The drawing under review shows one solid part. Ordinate dimensions are in mm from its lowest x, y, z. Give positions to 0.01 mm unless a question says otherwise; leave off trailing zeros. Write each loop counter-clockwise with the first axis right and the second up, starting at its lowest first coordinate (ties: lowest second). Pieces come first, ordered by that corner, then holes. Notation, with made-up numbers: M 67,8 L 117,8 A16 ccw 117,14 Z; hole C 42.25,30.5 d5. An arc over 180 degrees is marked long. Write item = value, one per line. Start each with the question number.
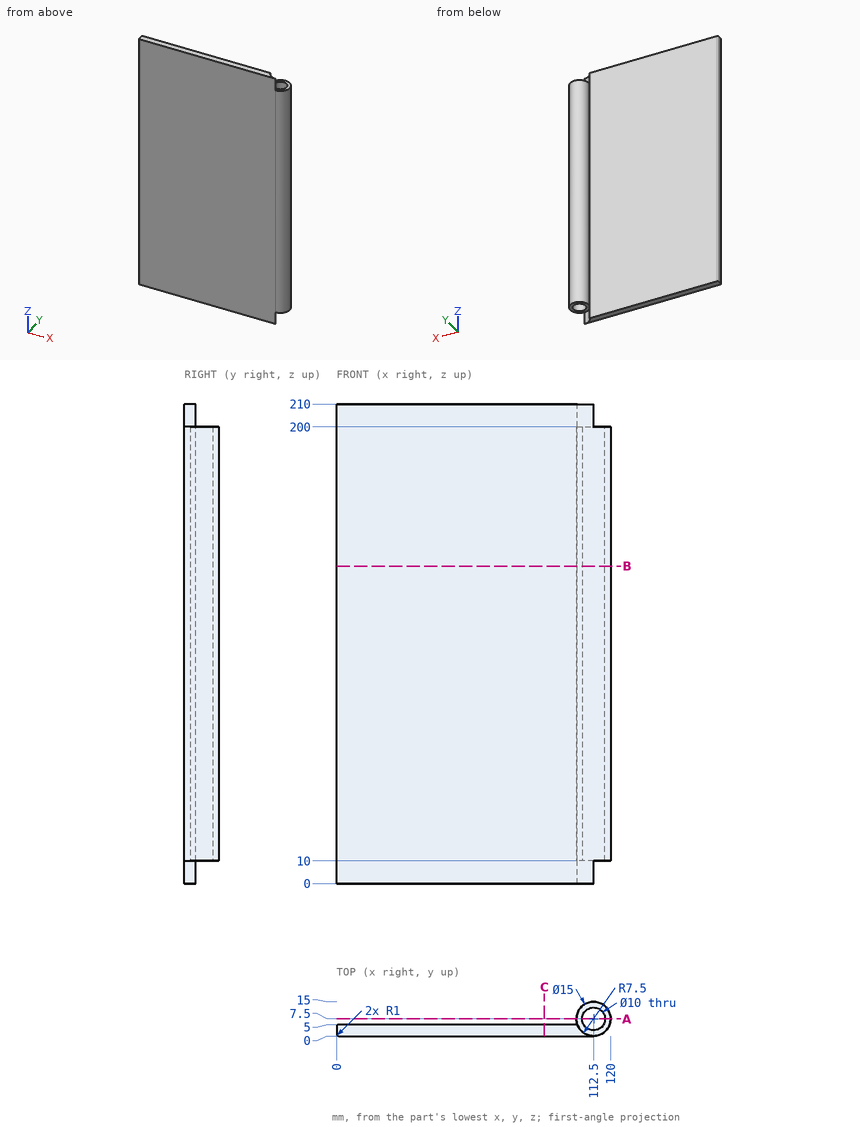
Item 1: We need section C-C, the plane x = 91. Write out the cut boundary in (y, z).
Item 2: Clearance check with flat-ended pins moving along their axes: P1, Ø1.5, axis at y = 13, z = 90, coming from the +X side; P2, Ø6, axis at x = 93, z = 79, coming from the +Y side. State where each tip first meets the part, or that it passes through.
Item 3: To check wall thickness, follow probe 1 along Y at (x, z) = (112.5, 130); probe 2 along X at (y, z) = (4.75, 196); probe 3 along X at (y, z) = (9.5, 48.5). State the ranges of each line that lie inside material, in increasing order. Write a range as [from, to].
Item 4: We need section A-A, the plane y = 7.5. Write out the cut boundary in (x, z).
Item 5: We need section B-B, the plane z = 139. Write out the cut boundary in (x, y).
Worked out:
q1.outline = M 0,0 L 5,0 L 5,210 L 0,210 Z
q2.P1 = 118.3
q2.P2 = 5
q3.probe_1 = [0, 2.5], [12.5, 15]
q3.probe_2 = [0.34, 108.32], [116.68, 119.48]
q3.probe_3 = [105.27, 107.92], [117.08, 119.73]
q4.outline = M 105,10 L 107.5,10 L 107.5,200 L 105,200 Z; M 117.5,10 L 120,10 L 120,200 L 117.5,200 Z
q5.outline = M 0,1 A1 ccw 1,0 L 112.5,0 A7.5 ccw long 105.43,5 L 1,5 A1 ccw 0,4 Z; hole C 112.5,7.5 d10
